Can you work these out from the model? Positions are in its coordinate system, mm. A direction names the side the tool comes from. Round coordinates to 2 decimals unless told otherwise and drop trailing zeros. Write each loop counter-clockwise with the first axis right and the second up, starting at its lowest first coordinate (ties: lowest second). Pieces come first, ordered by that corner, then holes. Notation, with made-up numbers: (-4.75, 33) - (54.25, 33) arc R22 ccw to (54.25, 61) - close; hole circle Ø11 at (61, -22.75). An arc over 180 degrees is marked (long way). One line per item, written item: value. Start each with the question number.
(1) I'm going to push flat-ended pins straight in: pin 1 Ø8 at (x, z) = (60.5, 5.5) entering from -Y; pin 2 Ø7 at (x, z) = (-20, -2.5) entering from +Y; pin 3 Ø24 at (x, y) = (51.5, 18.5) entering from -Z; pin 4 Ø5 at (x, z) = (54, 4.5) entering from +Y. Where does each tip first touch, or does it pass through?
(2) If I drill on L1, parallel to Y at x = -2, z = 15; L2, parallel to Y at x = 37, z = 4; L3, parallel to Y at x = 70, z = 5, over which ranges is the centre line in solid material (lowest first)? Write a range as from..to.
(3) Thinking about a two-plate mould opening in Z: for faces 1 (the face through (-26, -9, -9)), 2 (the face through (-22.93, 39.05, 11.85)), 3 (the face through (-28, -9, 5)), which applies, +Z half, -Z half, draft (parallel to the pull), parting line (faces both ways), or undercut?
(4) I want a section at A-A on x = -20. List the corners of the cut face in (y, z) for me, plus the area to 3 significant figures.
(5) I want a section at D-D on y = 38. Give the number of separate pieces and of enclosed holes in the cut face, plus the area to 3 significant figures.
(6) I want a section at B-B on x = 70. List the corners of the cut face in (y, z) for me, plus the area to 3 significant figures.
(7) On a 3-axis mill with a long thin cutter (end or side, diameter ignored), from which of +Z, -Z, +X, -X, +Y, -Y can I reach the whole of each face in a straight line? I mean faces 4 (the face through (81.99, 27.15, 5.07)), 5 (the face through (54, 0, 5)), 6 (the face through (-14, -5.5, 5)). Say none if no direction works.
(8) I want a section at C-C on z = 5. List the corners of the cut face in (x, y) for me, plus the area to 3 significant figures.
from build123d import *
from build123d.topology import SkipClean

# Parameters (mm, degrees)
SKETCH_1_W             = 85
SKETCH_1_H             = 30
EXTRUDE_1_DEPTH        = 10
EXTRUDE_2_DEPTH        = 10
EXTRUDE_2_DEPTH_BACK   = 20
SKETCH_3_W             = 8
SKETCH_3_H             = 30
SKETCH_2_R             = 8.5
CUT_EXTRUDE_1_DEPTH    = 10
SKETCH_5_W             = 8
SKETCH_5_H             = 30
EXTRUDE_3_DEPTH        = 12.5
SKETCH_6_W             = 30
SKETCH_6_H             = 7
EXTRUDE_4_DEPTH        = 28
CUT_EXTRUDE_2_REACH    = 99.115
SKETCH_7_R             = 3
FILLET_1_R             = 5
FILLET_1_OF_MIRROR_1_R = 5
FILLET_2_DEPTH         = 30
FILLET_3_DEPTH         = 30
FILLET_4_DEPTH         = 10
FILLET_START           = -9.709779072
FILLET_4_2_DEPTH       = 49.419558144
FILLET_START_2         = -11
FILLET_4_3_DEPTH       = 32
FILLET_START_3         = -10
FILLET_4_4_DEPTH       = 30
FILLET_6_R             = 10


with BuildPart() as part:
    # Sketch 1 → Extrude 1 (new body)
    with BuildSketch(Plane.XY):
        with Locations((42.5, 15)):
            Rectangle(SKETCH_1_W, SKETCH_1_H)
    extrude(amount=EXTRUDE_1_DEPTH)

    # Sketch 2 → Cut-Extrude 1 (cut)
    with BuildSketch(Plane(origin=(0, 0, 0), x_dir=(-1, 0, 0), z_dir=(0, 0, -1))):
        with Locations((-70, 15)):
            Circle(SKETCH_2_R)
    extrude(amount=-CUT_EXTRUDE_1_DEPTH, mode=Mode.SUBTRACT)



with BuildPart() as body_2:
    # Sketch 3 → Extrude 2 (new, two sides: drawn at the far end of the back side and taken through both)
    with BuildSketch(Plane.XY.offset(10).offset(-EXTRUDE_2_DEPTH_BACK)):
        with Locations((4, 15)):
            Rectangle(SKETCH_3_W, SKETCH_3_H)
    extrude(amount=EXTRUDE_2_DEPTH + EXTRUDE_2_DEPTH_BACK)


with BuildPart() as part_1:
    add(part.part)

    add(body_2.part)  # Extrude 3 merges body 2
    # Sketch 5 → Extrude 3 (add)
    with BuildSketch(Plane(origin=(0, 30, 0), x_dir=(1, 0, 0), z_dir=(0, 1, 0))):
        with Locations((4, -5)):
            Rectangle(SKETCH_5_W, SKETCH_5_H)
    extrude_3 = extrude(amount=EXTRUDE_3_DEPTH)

    # Sketch 6 → Extrude 4 (add)
    with BuildSketch(Plane.ZY):
        with Locations((5, 39)):
            Rectangle(SKETCH_6_W, SKETCH_6_H)
    extrude_4 = extrude(amount=EXTRUDE_4_DEPTH)

    # Sketch 7 → Cut-Extrude 2 (cut, up to next)
    with BuildSketch(Plane(origin=(0, 42.5, 0), x_dir=(1, 0, 0), z_dir=(0, 1, 0)), mode=Mode.PRIVATE) as cut_extrude_2_sk1:
        with Locations(Location((-20, 2.5, 0), (0, 0, 270))):
            Circle(SKETCH_7_R)
    cut_extrude_2_tool1 = extrude(cut_extrude_2_sk1.sketch, amount=-CUT_EXTRUDE_2_REACH, mode=Mode.PRIVATE) & part_1.part
    # Sketch 7 → Cut-Extrude 2 (cut, up to next)
    with BuildSketch(Plane(origin=(0, 42.5, 0), x_dir=(1, 0, 0), z_dir=(0, 1, 0)), mode=Mode.PRIVATE) as cut_extrude_2_sk2:
        with Locations(Location((-20, -12.5, 0), (0, 0, 270))):
            Circle(SKETCH_7_R)
    cut_extrude_2_tool2 = extrude(cut_extrude_2_sk2.sketch, amount=-CUT_EXTRUDE_2_REACH, mode=Mode.PRIVATE) & part_1.part
    cut_extrude_2_1 = cut_extrude_2_tool1.solids().sort_by_distance((-20, 42.5, -2.5))[0]
    add(cut_extrude_2_1, mode=Mode.SUBTRACT)
    cut_extrude_2_2 = cut_extrude_2_tool2.solids().sort_by_distance((-20, 42.5, 12.5))[0]
    add(cut_extrude_2_2, mode=Mode.SUBTRACT)
    cut_extrude_2 = cut_extrude_2_1 + cut_extrude_2_2  # Cut-Extrude 2 as one shape, for the pattern or mirror that repeats it

    # Fillet 1
    fillet_1_edges = [part_1.edges().sort_by_distance(p)[0] for p in [
        (8, 42.5, 5),
        (-28, 39, -10),
        (-28, 39, 20),
    ]]
    fillet(fillet_1_edges, radius=FILLET_1_R)

    # Mirror 1: Extrude 3, Extrude 4, Cut-Extrude 2 across plane
    add(extrude_3.mirror(Plane.ZX.offset(15)))
    add(extrude_4.mirror(Plane.ZX.offset(15)))
    add(cut_extrude_2.mirror(Plane.ZX.offset(15)), mode=Mode.SUBTRACT)

    # Fillet 1 of Mirror 1
    fillet_1_of_mirror_1_edges = [part_1.edges().sort_by_distance(p)[0] for p in [
        (8, -12.5, 5),
        (-28, -9, -10),
        (-28, -9, 20),
    ]]
    fillet(fillet_1_of_mirror_1_edges, radius=FILLET_1_OF_MIRROR_1_R)

    # Fillet 2: read off the stored shape, not the designer's step
    # Fillet 2 outline → Fillet 2 (add)
    with BuildSketch(Plane(origin=(0, 0, 0), x_dir=(1, 0, 0), z_dir=(0, 1, 0))):
        with BuildLine():
            add(Edge.make_bspline(
                [(33.980762114, -10), (13.773502692, -10), (8, -20)],
                knots=[0, 0, 0, 1, 1, 1], degree=2, weights=[1, 0.866025404, 1]))
            Line((33.980762114, -10), (8, -10))
            Line((8, -10), (8, -20))
        make_face()
    extrude(amount=FILLET_2_DEPTH)

    # Fillet 3: read off the stored shape, not the designer's step
    # Fillet 3 outline → Fillet 3 (add)
    with BuildSketch(Plane(origin=(0, 0, 0), x_dir=(1, 0, 0), z_dir=(0, 1, 0))):
        with BuildLine():
            Line((8, 0), (33.980762114, 0))
            add(Edge.make_bspline(
                [(33.980762114, 0), (13.773502692, 0), (8, 10)],
                knots=[0, 0, 0, 1, 1, 1], degree=2, weights=[1, 0.866025404, 1]))
            Line((8, 10), (8, 0))
        make_face()
    extrude(amount=FILLET_3_DEPTH)

    # Fillet 4: read off the stored shape, not the designer's step
    # Fillet 4 outline → Fillet 4 (add)
    with BuildSketch(Plane.XY):
        with BuildLine():
            ThreePointArc((6.458305444, -11.111111111), (19.217629145, -2.881570914), (34.124748995, 0))
            Line((34.124748995, 0), (8, 0))
            Line((8, 0), (8, -7.5))
            ThreePointArc((8, -7.5), (7.598452306, -9.463220922), (6.458305444, -11.111111111))
        make_face()
        with BuildLine():
            ThreePointArc((34.124748995, 30), (19.217629145, 32.881570914), (6.458305444, 41.111111111))
            ThreePointArc((6.458305444, 41.111111111), (7.598452306, 39.463220922), (8, 37.5))
            Line((8, 37.5), (8, 30))
            Line((8, 30), (34.124748995, 30))
        make_face()
    extrude(amount=FILLET_4_DEPTH)

    # Fillet 4 2 outline → Fillet 4 2 (add)
    with BuildSketch(Plane(origin=(0, 0, 0), x_dir=(1, 0, 0), z_dir=(0, 1, 0)).offset(FILLET_START)):
        with BuildLine():
            add(Edge.make_bspline(
                [(33.980762114, -10), (13.773502692, -10), (8, -20)],
                knots=[0, 0, 0, 1, 1, 1], degree=2, weights=[1, 0.866025404, 1]))
            Line((33.980762114, -10), (8, -10))
            Line((8, -10), (8, -20))
        make_face()
        with BuildLine():
            Line((8, 0), (33.980762114, 0))
            add(Edge.make_bspline(
                [(33.980762114, 0), (13.773502692, 0), (8, 10)],
                knots=[0, 0, 0, 1, 1, 1], degree=2, weights=[1, 0.866025404, 1]))
            Line((8, 10), (8, 0))
        make_face()
    extrude(amount=FILLET_4_2_DEPTH)

    # Fillet 4 3 outline → Fillet 4 3 (cut)
    with SkipClean():  # the faces are left unmerged after this step: merging them gives an invalid solid
        with BuildSketch(Plane.XY.offset(FILLET_START_2)):
            with BuildLine():
                Line((35, 0), (34.124748995, 0))
                ThreePointArc((34.124748995, 0), (20.189341563, -2.505941541), (7.99999995, -9.709779014))
                ThreePointArc((7.99999995, -9.709779014), (7.220027604, -10.400405968), (6.458305444, -11.111111111))
                Line((6.458305444, -11.111111111), (5, -12.507707754))
                Line((5, -12.507707754), (5, -13))
                Line((5, -13), (35, -13))
                Line((35, -13), (35, 0))
            make_face()
            with BuildLine():
                Line((34.124748995, 30), (35, 30))
                Line((35, 30), (35, 43))
                Line((35, 43), (5, 43))
                Line((5, 43), (5, 42.507707754))
                Line((5, 42.507707754), (6.458305444, 41.111111111))
                ThreePointArc((6.458305444, 41.111111111), (7.220027604, 40.400405968), (7.99999995, 39.709779014))
                ThreePointArc((7.99999995, 39.709779014), (20.189341563, 32.505941541), (34.124748995, 30))
            make_face()
        extrude(amount=FILLET_4_3_DEPTH, mode=Mode.SUBTRACT)
    add(part_1.part.scale(1), mode=Mode.REPLACE)  # the faces are merged on a copy

    # Fillet 4 4 outline → Fillet 4 4 (add)
    with BuildSketch(Plane.XY.offset(FILLET_START_3)):
        with BuildLine():
            ThreePointArc((6.458305444, -11.111111111), (7.220027604, -10.400405968), (7.99999995, -9.709779014))
            Line((7.99999995, -9.709779014), (8, -7.5))
            ThreePointArc((8, -7.5), (7.598452306, -9.463220922), (6.458305444, -11.111111111))
        make_face()
        with BuildLine():
            Line((8, 37.5), (7.99999995, 39.709779014))
            ThreePointArc((7.99999995, 39.709779014), (7.220027604, 40.400405968), (6.458305444, 41.111111111))
            ThreePointArc((6.458305444, 41.111111111), (7.598452306, 39.463220922), (8, 37.5))
        make_face()
    extrude(amount=FILLET_4_4_DEPTH)

    # Fillet 6
    fillet_6_edges = [part_1.edges().sort_by_distance(p)[0] for p in [
        (85, 0, 5),
        (85, 30, 5),
    ]]
    fillet(fillet_6_edges, radius=FILLET_6_R)


solid = part_1.part
Established:
1. pin 1: y = 0
1. pin 2: y = 42.5
1. pin 3: z = 0
1. pin 4: y = 30
2. L1: -12.5..-5.5, 35.5..42.5
2. L2: 0..30
2. L3: 0..6.5, 23.5..30
3. face 1: -Z half
3. face 2: undercut
3. face 3: draft
4. outline: (-12.5, -10) - (-5.5, -10) - (-5.5, -5.5) - (-12.5, -5.5) - close; (-12.5, 0.5) - (-5.5, 0.5) - (-5.5, 9.5) - (-12.5, 9.5) - close; (-12.5, 15.5) - (-5.5, 15.5) - (-5.5, 20) - (-12.5, 20) - close; (35.5, -10) - (42.5, -10) - (42.5, -5.5) - (35.5, -5.5) - close; (35.5, 0.5) - (42.5, 0.5) - (42.5, 9.5) - (35.5, 9.5) - close; (35.5, 15.5) - (42.5, 15.5) - (42.5, 20) - (35.5, 20) - close
4. area: 252 mm2
5. separate pieces: 1
5. enclosed holes: 2
5. area: 1,070 mm2
6. outline: (0, 0) - (6.5, 0) - (6.5, 10) - (0, 10) - close; (23.5, 0) - (30, 0) - (30, 10) - (23.5, 10) - close
6. area: 130 mm2
7. face 4: +Z, -Z, +X, +Y
7. face 5: +Z, -Z, +X, -Y
7. face 6: +Z, -Z, -X
8. outline: (-28, -12.5) - (3, -12.5) arc R5 ccw to (6.46, -11.11) arc R40 cw to (34.12, 0) - (75, 0) arc R10 ccw to (85, 10) - (85, 20) arc R10 ccw to (75, 30) - (34.12, 30) arc R40 cw to (6.46, 41.11) arc R5 ccw to (3, 42.5) - (-28, 42.5) - (-28, 35.5) - (0, 35.5) - (0, -5.5) - (-28, -5.5) - close; hole circle Ø17 at (70, 15)
8. area: 3,020 mm2
